```python
from build123d import *

# Parameters (mm, degrees)
F0_R     = 1.5875
F1_DEPTH = 25.4
F0_W     = 12.7
F0_H     = 38.608
F2_DEPTH = 6.35
F3_F1_R  = 1.27
F3_F2_R  = 1.27


with BuildPart() as f1:
    # F0 (on Top) → F1 (new body)
    with BuildSketch(Plane.XY):
        Polygon((19.05, 0), (19.05, 19.304), (-19.05, 19.304), (-19.05, -19.304), (19.05, -19.304), align=None)
        with Locations((-14.605, -10.414)):
            Circle(F0_R, mode=Mode.SUBTRACT)
        with Locations((14.605, -10.414)):
            Circle(F0_R, mode=Mode.SUBTRACT)
        with Locations((-14.605, 10.414)):
            Circle(F0_R, mode=Mode.SUBTRACT)
        with Locations((14.605, 10.414)):
            Circle(F0_R, mode=Mode.SUBTRACT)
    extrude(amount=F1_DEPTH)

    # F0 (on Top) → F2 (join)
    with BuildSketch(Plane.XY):
        with Locations((-25.4, 0)):
            Rectangle(F0_W, F0_H)
        with BuildLine():
            ThreePointArc((-27.78125, 12.954), (-25.4, 15.33525), (-23.01875, 12.954))
            Line((-23.01875, 12.954), (-23.01875, -12.954))
            ThreePointArc((-23.01875, -12.954), (-25.4, -15.33525), (-27.78125, -12.954))
            Line((-27.78125, -12.954), (-27.78125, 12.954))
        make_face(mode=Mode.SUBTRACT)
        Polygon((31.75, 19.304), (19.05, 19.304), (19.05, 0), (19.05, -19.304), (25.4, -19.304), (31.75, -19.304), align=None)
        with BuildLine():
            ThreePointArc((27.78125, -12.954), (27.0837980227, -14.6377980227), (25.4, -15.33525))
            ThreePointArc((25.4, -15.33525), (23.7162019773, -14.6377980227), (23.01875, -12.954))
            Line((23.01875, -12.954), (23.01875, 12.954))
            ThreePointArc((23.01875, 12.954), (25.4, 15.33525), (27.78125, 12.954))
            Line((27.78125, 12.954), (27.78125, -12.954))
        make_face(mode=Mode.SUBTRACT)
    extrude(amount=F2_DEPTH)

    # F3: fillet of radius 1.27 on 13 edges, made by hand

    # F3_f1
    f3_f1_edges = [f1.edges().sort_by_distance(p)[0] for p in [
        (-19.05, 0, 6.35),
        (19.05, 0, 6.35),
    ]]
    fillet(f3_f1_edges, radius=F3_F1_R)

    # F3_f2
    f3_f2_edges = [f1.edges().sort_by_distance(p)[0] for p in [
        (-19.05, -19.304, 16.51),
        (-19.05, 19.304, 16.51),
        (-31.75, 0, 6.35),
        (-31.75, -19.304, 3.175),
        (-31.75, 19.304, 3.175),
        (26.035, -19.304, 6.35),
        (19.05, -19.304, 16.51),
        (31.75, -19.304, 3.175),
        (31.75, 0, 6.35),
        (31.75, 19.304, 3.175),
        (26.035, 19.304, 6.35),
        (19.4219743879, 19.304, 6.7219743879),
        (19.4219743879, -19.304, 6.7219743879),
        (-19.4219743879, 19.304, 6.7219743879),
        (-19.4219743879, -19.304, 6.7219743879),
    ]]
    fillet(f3_f2_edges, radius=F3_F2_R)


solid = f1.part
```
Design review of the part built by this model. Coordinates are the model's own, in mm. A direction names the side the tool comes from. Coordinates: 2 decimals unless noted, no trailing zeros. Order: outer loops, then holes, each group sorted by start corner. A loop starts at its lowest first (then second) coordinate and runs counter-clockwise, first axis right, second up. Notation, with made-up numbers: (-34.75, 37.5) -> (5.25, 37.5) arc R16 cw to (5.25, 64.5) -> close; hole circle Ø4 at (-15.75, -23). An arc over 180 degrees is marked (long way). One line per item, written item: value. Start each with the question number.
Q1. Tool access review of faces 4 (the cylindrical face through (18.67, 18.94, 16.63)), 5 (the cylindrical face through (-25.452, 15.335, 3.131)), 6 (the flat face through (19.05, 0, 16)), 7 (the flat face through (-29, 0, 6.35)): name each direction out of +Z, -Z, +X, -X, +Y, -Y from which nothing blocks a thin tool from reaching the whole face with its end or side.
Q2. Insertion check: pin 1 Ø3 at (x, z) = (-18, 10.5) entering from +Y; pin 2 Ø2 at (y, z) = (-12.5, 20.5) entering from +X; pin 3 Ø5 at (x, y) = (-27, 3.5) entering from +Z; pin 4 Ø8 at (y, z) = (-6, 11) entering from +X. Each pin has a flat end and moves straight along its axis. Give the tip position at first contact, or say it passes through.
Q3. For probe 1 along X at (y, z) = (7, 4.5); probe 2 along X at (y, z) = (-11, 7); probe 3 along X at (y, z) = (-2.5, 17.5), list the stretches that pass through material, from the lowest coordinate up.
Q4. Take a section at A-A, the plane x = -25.4. State the section outline as (y, z) points, then the cut area to 3 significant figures.
Q5. Take a section at C-C, the plane z = 8.75. Give the number of separate pieces and of enclosed holes in the cut face, then the cut area to 3 significant figures.
Q6. Take a section at B-B, the plane y = 8. State the section outline as (x, z) points.
Q7. Mouldability with a two-part tool opening along X and no side actions: class faces 1 (the cylindrical face through (15.338, 9.006, 12.522)), 2 (the cylindrical face through (-18.67, 18.94, 16.63)), 3 (the flat face through (31.75, 0, 3)) as pulls with the +X half, pulls with the -X half, needs draft (parallel to the pull), parting line crosses it, or undercut.
Values follow:
1. face 4: +Z, +X, +Y
1. face 5: +Z, -Z
1. face 6: +Z, +X, +Y, -Y
1. face 7: +Z, -X, +Y, -Y
2. pin 1: stops at y = 19.3
2. pin 2: stops at x = 19.05
2. pin 3: stops at z = 6.35
2. pin 4: stops at x = 19.21
3. probe 1: x = -31.75 to -27.78, -23.02 to 23.02, 27.78 to 31.75
3. probe 2: x = -19.21 to -16.08, -13.13 to 13.13, 16.08 to 19.21
3. probe 3: x = -19.05 to 19.05
4. outline: (-19.3, 0) -> (-15.34, 0) -> (-15.34, 6.35) -> (-18.03, 6.35) arc R1.27 ccw to (-19.3, 5.08) -> close; (15.34, 0) -> (19.3, 0) -> (19.3, 5.08) arc R1.27 ccw to (18.03, 6.35) -> (15.34, 6.35) -> close
4. area: 49.7 mm2
5. separate pieces: 1
5. enclosed holes: 4
5. area: 1,440 mm2
6. outline: (-31.75, 0) -> (-27.78, 0) -> (-27.78, 6.35) -> (-30.48, 6.35) arc R1.27 ccw to (-31.75, 5.08) -> close; (-23.02, 0) -> (23.02, 0) -> (23.02, 6.35) -> (20.32, 6.35) arc R1.27 cw to (19.05, 7.62) -> (19.05, 25.4) -> (-19.05, 25.4) -> (-19.05, 7.62) arc R1.27 cw to (-20.32, 6.35) -> (-23.02, 6.35) -> close; (27.78, 0) -> (31.75, 0) -> (31.75, 5.08) arc R1.27 ccw to (30.48, 6.35) -> (27.78, 6.35) -> close
7. face 1: undercut
7. face 2: pulls with the -X half
7. face 3: pulls with the +X half
